Design review of the part built by this model. Coordinates are the model's own, in mm. A direction names the side the tool comes from. Coordinates: 2 decimals unless noted, no trailing zeros. Loops run counter-clockwise (first coordinate to the right, second up) from the corner with the lowest first, then second, coordinate; pieces in that order, holes last. Notation, with made-up numbers: (78, -32.75) -> (134, -32.75) arc R8 ccw to (134, -24.75) -> close; hole circle Ø11 at (-29.5, 65). An arc over 180 degrees is marked (long way). Use a Markdown table: item, result. Add a question column.
Q1. Take a section at D-D on z = 4.35. Write out the cut boundary in (x, y).
Q2. Draft analysis for pull direction X (two halves, no side actions). For faces 1 (the face through (1.46, 2.28, 3.11)), 2 (the face through (16.267, 2.218, 0.436)), 3 (the face through (1, 0, 3)), 4 (the face through (1.232, 2.218, 0.436)), state which applies: pulls with the +X half, pulls with the -X half, needs draft (parallel to the pull), parting line crosses it, or undercut.
Q3. For probe 1 along X at (y, z) = (3.95, 2.5); probe 2 along X at (y, z) = (0.3, 1); probe 3 along Y at (x, z) = (11.5, 1.25), list the stretches that pass through material, from the lowest coordinate up.
Q4. Take a section at A-A on y = 0.85. Write out the cut boundary in (x, z).
Q5. For faces 5 (the face through (14.75, 1, 1)), 6 (the face through (17.5, 2, 3)), list the 3-axis set-ups (+Z, -Z, +X, -X, +Y, -Y) from which the entire face can be reached by the end or side of a thin tool; tool diameter is ignored.
Q6. Clearance check with flat-ended pins moving along their axes: pin 1 Ø1.2 at (y, z) = (0.5, 0.5) entering from -X; pin 2 Ø2.5 at (x, z) = (9.5, 3.5) entering from -Y. State where each tip first meets the part, or that it passes through.
Q7. Take a section at C-C on x = 15.25. Write out the cut boundary in (y, z).
Q8. Take a section at B-B on z = 2.5. Write out the cut boundary in (x, y), plus the area to 4 significant figures.
from build123d import *

# Parameters (mm, degrees)
SKETCH_1_W          = 17.5
SKETCH_1_H          = 4.5
EXTRUDE_1_DEPTH     = 5
SKETCH_2_R          = 1
CUT_EXTRUDE_1_DEPTH = 5.5
SKETCH_3_W          = 12
SKETCH_3_H          = 1.5
CUT_EXTRUDE_3_DEPTH = 6
CHAMFER_2_SIZE      = 2.5
CHAMFER_2_SIZE2     = 0.860819033


with BuildPart() as part:
    # Эскиз1 → Бобышка-Вытянуть1 (new body)
    with BuildSketch(Plane.XY):
        with Locations((8.75, 2.25)):
            Rectangle(SKETCH_1_W, SKETCH_1_H)
    extrude(amount=EXTRUDE_1_DEPTH)

    # Эскиз2 → Вырез-Вытянуть1 (cut, through all)
    with BuildSketch(Plane(origin=(0, 4.5, 0), x_dir=(1, 0, 0), z_dir=(0, 1, 0))):
        with Locations((2.25, -2.5)):
            Circle(SKETCH_2_R)
        with Locations((15.25, -2.5)):
            Circle(SKETCH_2_R)
    extrude(amount=-CUT_EXTRUDE_1_DEPTH, mode=Mode.SUBTRACT)

    # Эскиз3 → Вырез-Вытянуть3 (cut, through all)
    with BuildSketch(Plane.XY.offset(5)):
        with Locations((8.75, 0.75)):
            Rectangle(SKETCH_3_W, SKETCH_3_H)
    extrude(amount=-CUT_EXTRUDE_3_DEPTH, mode=Mode.SUBTRACT)

    # Фаска2
    chamfer_2_edges = [part.edges().sort_by_distance(p)[0] for p in [
        (17.5, 2.25, 0),
        (0, 2.25, 0),
    ]]
    chamfer_2_side = [part.faces().sort_by_distance(p)[0] for p in [
        (8.75, 2.694444444, 0),
    ]]
    chamfer(chamfer_2_edges, length=CHAMFER_2_SIZE, length2=CHAMFER_2_SIZE2, reference=chamfer_2_side[0])


solid = part.part
Answer list:
| question | item | result |
|---|---|---|
| 1 | outline | (0, 0) -> (2.75, 0) -> (2.75, 1.5) -> (14.75, 1.5) -> (14.75, 0) -> (17.5, 0) -> (17.5, 4.5) -> (0, 4.5) -> close |
| 2 | face 1 | undercut |
| 2 | face 2 | pulls with the +X half |
| 2 | face 3 | needs draft |
| 2 | face 4 | pulls with the -X half |
| 3 | probe 1 | 0 to 1.25, 3.25 to 14.25, 16.25 to 17.5 |
| 3 | probe 2 | 0 to 2.75, 14.75 to 17.5 |
| 3 | probe 3 | 1.5 to 4.5 |
| 4 | outline | (0, 0.86) -> (2.5, 0) -> (2.75, 0) -> (2.75, 1.63) arc R1 cw (long way) to (2.75, 3.37) -> (2.75, 5) -> (0, 5) -> close; (14.75, 0) -> (15, 0) -> (17.5, 0.86) -> (17.5, 5) -> (14.75, 5) -> (14.75, 3.37) arc R1 cw (long way) to (14.75, 1.63) -> close |
| 5 | face 5 | +Z, -Z, -Y |
| 5 | face 6 | +Z, -Z, +X, +Y, -Y |
| 6 | pin 1 | x = 0 |
| 6 | pin 2 | y = 1.5 |
| 7 | outline | (0, 0.09) -> (4.5, 0.09) -> (4.5, 1.5) -> (0, 1.5) -> close; (0, 3.5) -> (4.5, 3.5) -> (4.5, 5) -> (0, 5) -> close |
| 8 | outline | (0, 0) -> (1.25, 0) -> (1.25, 4.5) -> (0, 4.5) -> close; (3.25, 1.5) -> (14.25, 1.5) -> (14.25, 4.5) -> (3.25, 4.5) -> close; (16.25, 0) -> (17.5, 0) -> (17.5, 4.5) -> (16.25, 4.5) -> close |
| 8 | area | 44.25 mm² |
